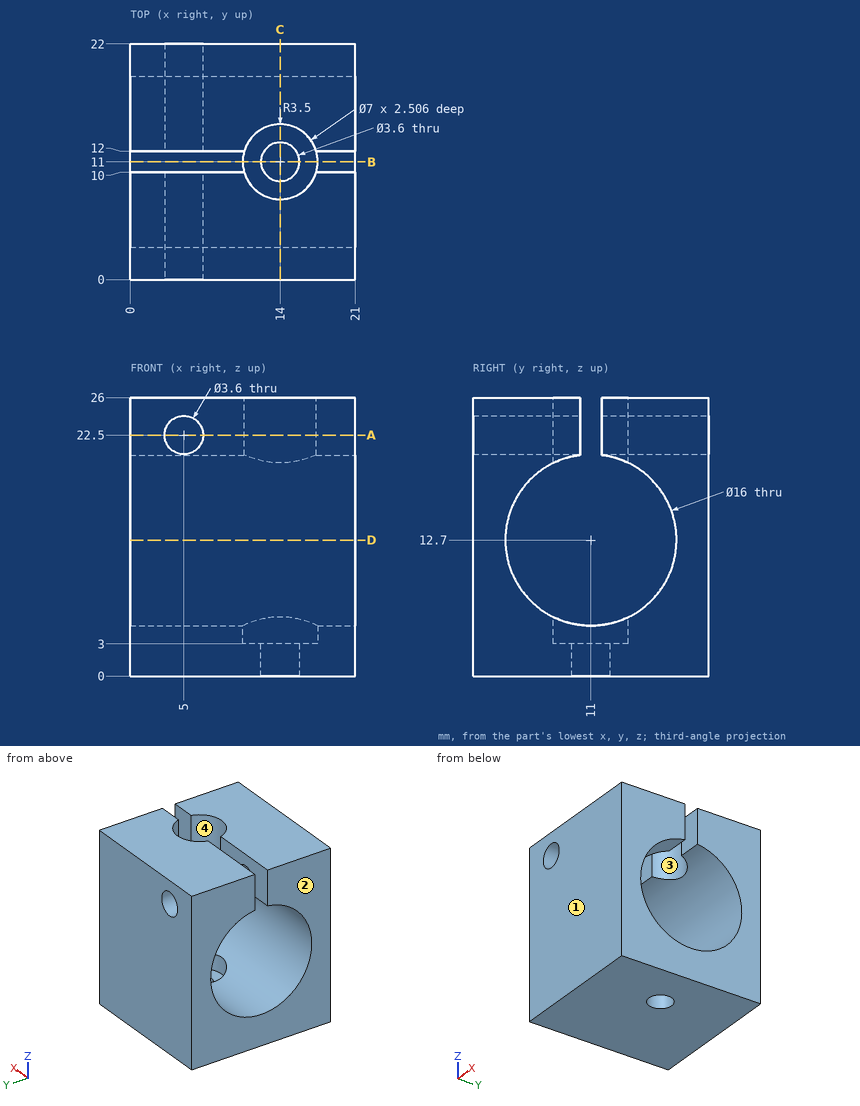
Check sheet for the drawn part. Datum: minimum x, y, z corner. Units: mm. Round coordinates to 2 decimals unless told otherwise and drop trailing zeros. Write each loop counter-clockwise with the first axis right and the second up, starting at its lowest first coordinate (ties: lowest second). Pieces come first, ordered by that corner, then holes. Notation, with made-up numbers: (-23.75, -30) -> (-19.75, -30) arc R23 cw to (-19.75, 5) -> close; hole circle Ø10 at (-9.75, 71). An arc over 180 degrees is marked (long way). One line per item, written item: value. Start each with the question number.
(1) Cross-section at A-A, the plane z = 22.5. Record the cut outline in (x, y).
(2) Scan lines: line 1 (Z direction, x = 5, y = 14.5); line 2 (Y direction, x = 5.75, z = 12.75); line 3 (Z direction, x = 5, y = 17.5) (1 decimal). Record each from-to range of solid material in increasing order. Write a range as [from, to].
(3) Cross-section at D-D, the plane z = 12.7. Record the cut outline in (x, y), and give its area (3 significant figures).
(4) Cross-section at B-B, the plane y = 11. Record the cut outline in (x, z).
(5) Cross-section at C-C, the plane x = 14. Record the cut outline in (y, z).
(6) Draft check along X on the marked faces 1, 2, 3 and 4. Enter one of: +X half, -X half, draft (parallel to the pull), parting line (faces both ways), or undercut.
Answer:
1. outline: (0, 0) -> (3.2, 0) -> (3.2, 10) -> (0, 10) -> close; (0, 12) -> (3.2, 12) -> (3.2, 22) -> (0, 22) -> close; (6.8, 0) -> (21, 0) -> (21, 10) -> (17.35, 10) arc R3.5 cw to (10.65, 10) -> (6.8, 10) -> close; (6.8, 12) -> (10.65, 12) arc R3.5 cw to (17.35, 12) -> (21, 12) -> (21, 22) -> (6.8, 22) -> close
2. line 1: [0, 5.51], [19.89, 20.7], [24.3, 26]
2. line 2: [0, 3], [19, 22]
2. line 3: [0, 8], [17.4, 20.7], [24.3, 26]
3. outline: (0, 0) -> (21, 0) -> (21, 3) -> (0, 3) -> close; (0, 19) -> (21, 19) -> (21, 22) -> (0, 22) -> close
3. area: 126 mm²
4. outline: (0, 0) -> (12.2, 0) -> (12.2, 3) -> (10.5, 3) -> (10.5, 4.7) -> (0, 4.7) -> close; (15.8, 0) -> (21, 0) -> (21, 4.7) -> (17.5, 4.7) -> (17.5, 3) -> (15.8, 3) -> close
5. outline: (0, 0) -> (9.2, 0) -> (9.2, 3) -> (7.5, 3) -> (7.5, 5.51) arc R8 cw to (7.5, 19.89) -> (7.5, 26) -> (0, 26) -> close; (12.8, 0) -> (22, 0) -> (22, 26) -> (14.5, 26) -> (14.5, 19.89) arc R8 cw to (14.5, 5.51) -> (14.5, 3) -> (12.8, 3) -> close
6. face 1: draft
6. face 2: -X half
6. face 3: undercut
6. face 4: undercut
